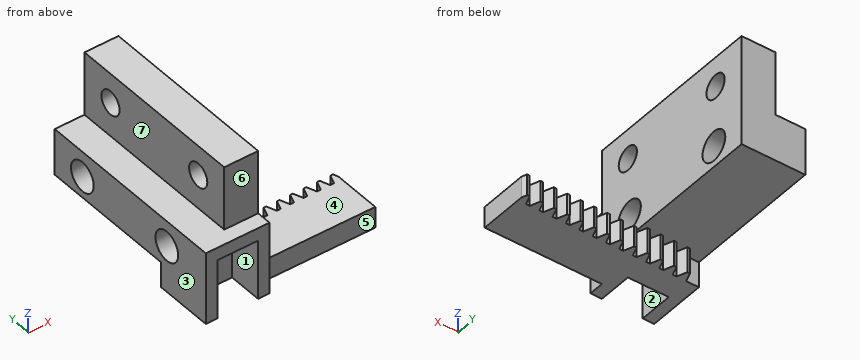
```python
from build123d import *

# Parameters (mm, degrees)
BLANKSKE_W                 = 40
BLANKSKE_H                 = 12.5
BLANK_DEPTH                = 5
TOOTHCUTSIM_DEPTH          = 43.20485754
TEETHCUTS_COUNT            = 14
TEETHCUTS_PITCH            = 3.14159265
MOVE_FACE1_BY              = 0.44
SKETCH1_W                  = 15
SKETCH1_H                  = 43
BOSS_EXTRUDE1_DEPTH        = 12
F_7_0_7_DIAMETER_HOLE1_D   = 7
SKETCH6_W                  = 2.7
SKETCH6_H                  = 17
BOSS_EXTRUDE2_DEPTH        = 3.5
SKETCH7_W                  = 8
SKETCH7_H                  = 43
BOSS_EXTRUDE3_DEPTH        = 15
F_5_6_5_6_DIAMETER_HOLE1_D = 5.6
MOVE_FACE2_BY              = 3
SKETCH11_W                 = 9.6
SKETCH11_H                 = 14
CUT_EXTRUDE2_DEPTH         = 4.5
SKETCH12_W                 = 9.6
SKETCH12_H                 = 3
BOSS_EXTRUDE4_DEPTH        = 3.5
MOVE_FACE3_BY              = 1


with BuildPart() as part:
    # BlankSke → Blank (new body)
    with BuildSketch(Plane.XY):
        with Locations((20, 6.25)):
            Rectangle(BLANKSKE_W, BLANKSKE_H)
    extrude(amount=-BLANK_DEPTH)

    # TooCutSkeSim → ToothCutSim (cut, through all)
    with BuildSketch(Plane.XY):
        Polygon((0.44443537, 10.25), (-0.44443537, 10.25), (-1.272613241, 12.5254), (1.272613241, 12.5254), align=None)
    toothcutsim = extrude(amount=-TOOTHCUTSIM_DEPTH, mode=Mode.SUBTRACT)

    # TeethCuts: ToothCutSim ×14
    with Locations(*[(i * TEETHCUTS_PITCH, 0, 0) for i in range(1, TEETHCUTS_COUNT)]):
        add(toothcutsim, mode=Mode.SUBTRACT)

    # Move Face1: a face moved inward by 0.44
    extrude(part.faces().sort_by_distance((0, 5.125, -2.5))[0], amount=MOVE_FACE1_BY, dir=(1, 0, 0), mode=Mode.SUBTRACT)

    # Sketch1 → Boss-Extrude1 (add)
    with BuildSketch(Plane(origin=(0, 0, 0), x_dir=(-1, 0, 0), z_dir=(0, 0, -1))):
        with Locations((-4.94, 21.5)):
            Rectangle(SKETCH1_W, SKETCH1_H)
    extrude(amount=-BOSS_EXTRUDE1_DEPTH)

    # Ø7.0 (7) Diameter Hole1 (through all)
    with Locations(Plane.ZY.offset(2.56)):
        with Locations((6, 34.5), (6, 8.5)):
            Hole(F_7_0_7_DIAMETER_HOLE1_D / 2)

    # Sketch6 → Boss-Extrude2 (add)
    with BuildSketch(Plane.XZ):
        with Locations((-1.21, 3.5)):
            Rectangle(SKETCH6_W, SKETCH6_H)
        with Locations((11.09, 3.5)):
            Rectangle(SKETCH6_W, SKETCH6_H)
    extrude(amount=BOSS_EXTRUDE2_DEPTH)

    # Sketch7 → Boss-Extrude3 (add)
    with BuildSketch(Plane.XY.offset(12)):
        with Locations((8.44, 21.5)):
            Rectangle(SKETCH7_W, SKETCH7_H)
    extrude(amount=BOSS_EXTRUDE3_DEPTH)

    # Ø5.6 (5.6) Diameter Hole1 (through all)
    with Locations(Plane(origin=(12.44, 0, 0), x_dir=(0, 0, -1), z_dir=(1, 0, 0))):
        with Locations((-20, 35), (-20, 8)):
            Hole(F_5_6_5_6_DIAMETER_HOLE1_D / 2)

    # Move Face2: a face moved outward by 3.0
    extrude(part.faces().sort_by_distance((0.44, 5.125, -2.5))[0], amount=MOVE_FACE2_BY, dir=(-1, 0, 0))

    # Sketch11 → Cut-Extrude2 (cut)
    with BuildSketch(Plane.XZ):
        with Locations((4.94, 2)):
            Rectangle(SKETCH11_W, SKETCH11_H)
    extrude(amount=-CUT_EXTRUDE2_DEPTH, mode=Mode.SUBTRACT)

    # Sketch12 → Boss-Extrude4 (add)
    with BuildSketch(Plane.XZ):
        with Locations((4.94, 10.5)):
            Rectangle(SKETCH12_W, SKETCH12_H)
    extrude(amount=BOSS_EXTRUDE4_DEPTH)

    # Move Face3: a face moved inward by 1.0
    extrude(part.faces().sort_by_distance((4.903765557, 27.042169716, 0))[0], amount=MOVE_FACE3_BY, dir=(0, 0, 1), mode=Mode.SUBTRACT)


solid = part.part
```
Geometry: final body of the model. Coordinates: model frame, mm. Face numbers are marked on the shaded views. A direction names the side the tool comes from. Coordinates: 2 decimals unless noted, no trailing zeros. Order: outer loops, then holes, each group sorted by start corner. A loop starts at its lowest first (then second) coordinate and runs counter-clockwise, first axis right, second up. Notation, with made-up numbers: (54, 13) -> (113, 13) arc R10 ccw to (113, 32) -> close; hole circle Ø6 at (-2.5, 87). An arc over 180 degrees is marked (long way). Write item = value, one per line.
(1) Cut plane C-C on z = 10.5. Return loops of the section in (x, y).
Solved:
outline = (-2.56, -3.5) -> (12.44, -3.5) -> (12.44, 43) -> (-2.56, 43) -> close
(2) Line query: line 1 (Y direction, x = 7.75, z = 20); line 2 (Y direction, x = 0, z = 6); line 3 (X direction, y = 24, z = 19). Output: solid intervals per line, ascending.
Solved:
line_1 = 0 to 5.2, 10.8 to 32.2, 37.8 to 43
line_2 = -3.5 to 5, 12 to 31, 38 to 43
line_3 = 4.44 to 12.44
(3) Pin query (flat end, axial travel): pin 1 Ø10 at (y, z) = (26.5, 12) entering from +X; pin 2 Ø0.5 at (x, z) = (27, -3) entering from +Y; pin 3 Ø4.5 at (x, y) = (5, 24.5) entering from -Z. Return the tip coordinate at first contact, or that it passes through.
Solved:
pin_1 = 12.44
pin_2 = 12.5
pin_3 = 1
(4) Cut plane D-D on z = 23.5. Return loops of the section in (x, y), plus the area to 3 significant figures.
Solved:
outline = (4.44, 0) -> (12.44, 0) -> (12.44, 43) -> (4.44, 43) -> close
area = 344 mm²
(5) Cut plane B-B on y = 39.5. Return loops of the section in (x, z), plus the area to 3 significant figures.
Solved:
outline = (-2.56, 1) -> (12.44, 1) -> (12.44, 27) -> (4.44, 27) -> (4.44, 12) -> (-2.56, 12) -> close
area = 285 mm²
(6) Cut plane A-A on z = 20. Return loops of the section in (x, y).
Solved:
outline = (4.44, 0) -> (12.44, 0) -> (12.44, 5.2) -> (4.44, 5.2) -> close; (4.44, 10.8) -> (12.44, 10.8) -> (12.44, 32.2) -> (4.44, 32.2) -> close; (4.44, 37.8) -> (12.44, 37.8) -> (12.44, 43) -> (4.44, 43) -> close
(7) Pull-direction query (X, two-part tool) for the marked faces 1, 2, 3 and 4; classes: pulls with the +X half, pulls with the -X half, needs draft (parallel to the pull), parting line crosses it, or undercut.
Solved:
face_1 = undercut
face_2 = undercut
face_3 = pulls with the -X half
face_4 = needs draft
(8) Access query for the marked faces 5, 6 and 7. Directions: +Z, -Z, +X, -X, +Y, -Y. A direction counts if a zero-diameter tool reaches every point of the face in a straight line with its end or side. Return the directions, or none.
Solved:
face_5 = +Z, -Z, +X, -Y
face_6 = +Z, +X, -X, -Y
face_7 = +Z, -X, +Y, -Y
